Work out the finished part from the listing and answer in its coordinate system (mm). A direction names the side the tool comes from. Coordinates: 2 decimals unless noted, no trailing zeros. Order: outer loops, then holes, each group sorted by start corner. A loop starts at its lowest first (then second) coordinate and runs counter-clockwise, first axis right, second up.
1. The part is cut by section B-B, the plane z = -296. Give the vertices of the cut face in (x, y), then the cut area to 3 significant figures.
2. The part is cut by section C-C, the plane y = 60. Give the vertices of the cut face in (x, z), then the cut area to 3 significant figures.
3. Find the intervals of material crossed by probe 1 along Y at (x, z) = (-22.5, -64.5); probe 2 along Z at (x, y) = (-24, 67.5), in increasing order.
4. Flat-ended cylindrical pins translate along their axes: pin 1 Ø13 at (x, y) = (-30, 68.5) entering from +Z; pin 2 Ø5 at (x, y) = (-10, 60.5) entering from -Z. Find the tip coordinate at first contact, or state that the pin passes through.
5. The part is cut by section A-A, the plane x = -29. Give the vertices of the cut face in (y, z), then the cut area to 3 significant figures.
6. A tool of negligible diameter and unlimited length cuts with its end or side. For faces 1 (the flat face through (-25, 64, -217)), 2 (the flat face through (-25, 25, 0)), 3 (the flat face through (-25, 64, -121)), from which of +Z, -Z, +X, -X, +Y, -Y can it reach the whole face along a straight path? Write none if from no direction.
Autodesk Inventor part; units mm, degrees
ref_plane "YZ Plane" through (0, 0, 0) normal (1, 0, 0) x (0, 1, 0)
ref_plane "XZ Plane" through (0, 0, 0) normal (0, 1, 0) x (-1, 0, 0)
ref_plane "XY Plane" through (0, 0, 0) normal (0, 0, 1) x (1, 0, 0)
sketch "Sketch1" plane through (0, 0, 0) normal (0, 1, 0) x (-1, 0, 0)
  line L0 (0, 0) -> (50.8, 0)
  line L1 (50.8, 0) -> (50.8, -334)
  line L2 (50.8, -334) -> (0, -334)
  line L3 (0, -334) -> (0, 0)
  dimension "d0" = 50.8
  dimension "d1" = 334
extrude "Extrusion1" add sketch "Sketch1" along normal blind 77
sketch "Sketch3" plane through (0, 0, 0) normal (1, 0, 0) x (0, 0, -1)
  line L0 (0, 77) -> (121, 77)
  line L1 (121, 77) -> (121, 51.2)
  line L2 (121, 51.2) -> (0, 51.2)
  line L3 (0, 51.2) -> (0, 77)
  line L4 (0, 77) -> (334, 77)
  line L5 (334, 77) -> (217, 77)
  line L6 (217, 77) -> (217, 51.2)
  line L7 (217, 51.2) -> (334, 51.2)
  line L8 (334, 51.2) -> (334, 77)
  point P0 (0, 0)
  dimension "d9" = 25.8
  dimension "d10" = 117
  dimension "d11" = 25.8
  dimension "d14" = 96
extrude "Extrusion2" cut sketch "Sketch3" against normal blind 52.8
properties part number "PiezaPuerta-1"
Geometry says:
1. outline: (-50.8, 0) - (0, 0) - (0, 51.2) - (-50.8, 51.2) - close
1. area: 2,600 mm2
2. outline: (-50.8, -217) - (0, -217) - (0, -121) - (-50.8, -121) - close
2. area: 4,880 mm2
3. probe 1: y = 0 to 51.2
3. probe 2: z = -217 to -121
4. pin 1: stops at z = -121
4. pin 2: stops at z = -217
5. outline: (0, -334) - (51.2, -334) - (51.2, -217) - (77, -217) - (77, -121) - (51.2, -121) - (51.2, 0) - (0, 0) - close
5. area: 19,600 mm2
6. face 1: -Z, +X, -X, +Y
6. face 2: +Z, +X, -X, +Y, -Y
6. face 3: +Z, +X, -X, +Y
